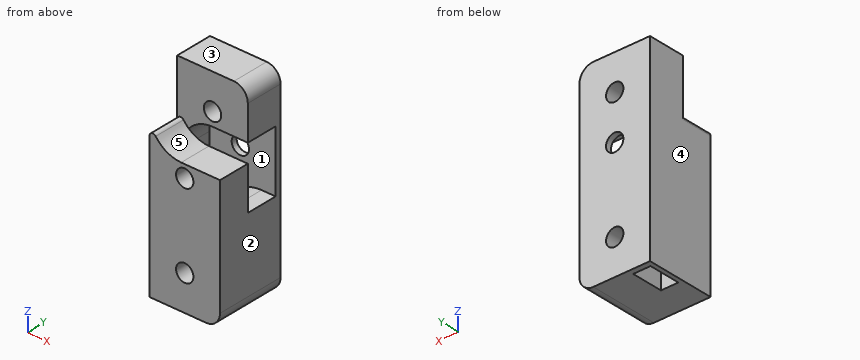
```python
from build123d import *

# Parameters (mm, degrees)
SKETCH1_W           = 20.32
SKETCH1_H           = 57.05
SKETCH1_R           = 2.5
BOSS_EXTRUDE1_DEPTH = 19.9
FILLET1_R           = 4
CUT_EXTRUDE1_DEPTH  = 9.136
SKETCH3_R           = 2.5
CUT_EXTRUDE2_DEPTH  = 20.9
CUT_EXTRUDE3_START  = -10.764
CUT_EXTRUDE3_DEPTH  = 9.136
FILLET2_R           = 1


with BuildPart() as part:
    # Sketch1 → Boss-Extrude1 (new body)
    with BuildSketch(Plane(origin=(0, 0, 0), x_dir=(1, 0, 0), z_dir=(0, 1, 0))):
        with Locations((0, 18.365)):
            Rectangle(SKETCH1_W, SKETCH1_H)
        Circle(SKETCH1_R, mode=Mode.SUBTRACT)
        with Locations((0, 36.73)):
            Circle(SKETCH1_R, mode=Mode.SUBTRACT)
    extrude(amount=BOSS_EXTRUDE1_DEPTH)

    # Fillet1
    fillet1_edges = [part.edges().sort_by_distance(p)[0] for p in [
        (10.16, 9.95, 10.16),
        (10.16, 9.95, -46.89),
    ]]
    fillet(fillet1_edges, radius=FILLET1_R)

    # Sketch2 → Cut-Extrude1 (cut)
    with BuildSketch(Plane.XZ):
        with BuildLine():
            Line((-1.016, -9.144), (10.16, -9.144))
            Line((10.16, -9.144), (10.16, 10.16))
            Line((10.16, 10.16), (-10.16, 10.16))
            Line((-10.16, 10.16), (-10.16, 0))
            ThreePointArc((-10.16, 0), (-7.481784407, -6.465784407), (-1.016, -9.144))
        make_face()
    extrude(amount=-CUT_EXTRUDE1_DEPTH, mode=Mode.SUBTRACT)

    # Sketch3 → Cut-Extrude2 (cut, through all)
    with BuildSketch(Plane(origin=(0, 19.9, 0), x_dir=(1, 0, 0), z_dir=(0, 1, 0))):
        with Locations((0, 12.73)):
            Circle(SKETCH3_R)
    extrude(amount=-CUT_EXTRUDE2_DEPTH, mode=Mode.SUBTRACT)

    # Sketch4 → Cut-Extrude3 (cut)
    with BuildSketch(Plane(origin=(0, 19.9, 0), x_dir=(1, 0, 0), z_dir=(0, 1, 0)).offset(CUT_EXTRUDE3_START)):
        with BuildLine():
            Line((0, 3.84), (10.16, 3.84))
            Line((10.16, 3.84), (10.16, 21.62))
            Line((10.16, 21.62), (6.11, 21.62))
            ThreePointArc((6.11, 21.62), (-0.961067812, 24.548932188), (-3.89, 31.62))
            Line((-3.89, 31.62), (-3.89, 46.89))
            Line((-3.89, 46.89), (-8.89, 46.89))
            Line((-8.89, 46.89), (-8.89, 12.73))
            ThreePointArc((-8.89, 12.73), (-6.286179285, 6.443820715), (0, 3.84))
        make_face()
    extrude(amount=CUT_EXTRUDE3_DEPTH, mode=Mode.SUBTRACT)

    # Fillet2
    fillet2_edges = [part.edges().sort_by_distance(p)[0] for p in [
        (-10.16, 4.568, 0),
    ]]
    fillet(fillet2_edges, radius=FILLET2_R)


solid = part.part
```
Read the model definition and answer for the solid it produces. Units are mm, in the model's axes. Face numbers are marked on the shaded views. A direction names the side the tool comes from. Coordinates: 2 decimals unless noted, no trailing zeros. Loops run counter-clockwise (first coordinate to the right, second up) from the corner with the lowest first, then second, coordinate; pieces in that order, holes last. Notation, with made-up numbers: (41.25, 19.5) - (69.25, 19.5) arc R35 ccw to (69.25, 51.5) - close; hole circle Ø5 at (-39.5, -9.75). An arc over 180 degrees is marked (long way). Answer in a Markdown table with one row per item.
1. Given pin 1 (4.5 mm diameter, centred on x = 5.5, y = 5.5, fed in from +Z); pin 2 (8 mm diameter, centred on x = -7.5, y = 9, fed in from +Z); pin 3 (12 mm diameter, centred on x = 6, z = -2.5, fed in from -Y); pin 4 (4 mm diameter, centred on x = 0, z = -12.73, fed in from +Y), each flat-ended and moving along its own axis, determine where each tip first touches the part or whether it passes through.
Conclusion:
| item | result |
|---|---|
| pin 1 | stops at z = -9.14 |
| pin 2 | stops at z = 10.16 |
| pin 3 | stops at y = 9.14 |
| pin 4 | passes through |
2. Which of the six approach directions +Z, -Z, +X, -X, +Y, -Y give full straight-line access (tool end or side, diameter ignored) to the marked faces 4 and 5?
Conclusion:
| item | result |
|---|---|
| face 4 | +Z, -Z, -X, +Y, -Y |
| face 5 | +Z, +X, -Y |
3. Straight lines are drawn through the part: line 1 (Z direction, x = 0, y = 19.5); line 2 (Z direction, x = 0, y = 2); line 3 (Y direction, x = -8.75, z = -44). For each, find the intervals that lie inside material, in ascending order.
Conclusion:
| item | result |
|---|---|
| line 1 | z = -46.89 to -39.23, -34.23 to -15.23, -10.23 to -2.5, 2.5 to 10.16 |
| line 2 | z = -46.89 to -39.23, -34.23 to -15.23, -10.23 to -9.14 |
| line 3 | y = 0 to 9.14, 18.27 to 19.9 |
4. Find section C-C, the plane z = 0. Write down the section's boundary in (x, y).
Conclusion:
| item | result |
|---|---|
| outline | (-10.16, 9.14) - (-2.5, 9.14) - (-2.5, 19.9) - (-10.16, 19.9) - close; (2.5, 9.14) - (10.16, 9.14) - (10.16, 19.9) - (2.5, 19.9) - close |
5. Find section D-D, the plane x = -5.75. Write down the section's boundary in (y, z).
Conclusion:
| item | result |
|---|---|
| outline | (0, -46.89) - (9.14, -46.89) - (9.14, -7.82) - (0, -7.82) - close; (9.14, -5.95) - (18.27, -5.95) - (18.27, -46.89) - (19.9, -46.89) - (19.9, 10.16) - (9.14, 10.16) - close |
6. Find section B-B, the plane z = -36.73. Write down the section's boundary in (x, y), then the cut area to 3 significant figures.
Conclusion:
| item | result |
|---|---|
| outline | (-10.16, 0) - (-2.5, 0) - (-2.5, 19.9) - (-10.16, 19.9) - close; (2.5, 0) - (10.16, 0) - (10.16, 19.9) - (2.5, 19.9) - close; hole (-8.89, 9.14) - (-3.89, 9.14) - (-3.89, 18.27) - (-8.89, 18.27) - close |
| area | 259 mm² |
7. Find section A-A, the plane y = 12.5. Write down the section's boundary in (x, z), then the cut area to 3 significant figures.
Conclusion:
| item | result |
|---|---|
| outline | (-10.16, -46.89) - (-8.89, -46.89) - (-8.89, -12.73) arc R8.89 cw to (0, -3.84) - (10.16, -3.84) - (10.16, 6.16) arc R4 ccw to (6.16, 10.16) - (-10.16, 10.16) - close; (-3.89, -46.89) - (6.16, -46.89) arc R4 ccw to (10.16, -42.89) - (10.16, -21.62) - (6.11, -21.62) arc R10 ccw to (-3.89, -31.62) - close; hole circle Ø5 at (0, -36.73); hole circle Ø5 at (0, 0) |
| area | 644 mm² |
8. Determine the mould class of the marked faces 1, 2 and 3 for opening direction X: +X half, -X half, draft (parallel to the pull), parting line (faces both ways), or undercut.
Conclusion:
| item | result |
|---|---|
| face 1 | undercut |
| face 2 | +X half |
| face 3 | draft |
